Can you work these out from the drawing? Everything is in mm from the part's minimum corner. Give positions to 0.01 mm unless a question says otherwise; leave off trailing zeros. Order: outer loops, then holes, each group sorted by start corner. A loop starts at its lowest first (then second) coordinate and runs counter-clockwise, first axis right, second up. Notation, with made-up numbers: M -37.75,47.25 L -9.75,47.25 A19 cw -9.75,69.25 Z; hole C 28.5,61.5 d7. An arc over 180 degrees is marked long. Use a Markdown table: item, result. Add a question column.
Item 1: Suppose I cut it at B-B on y = 12. Write out the boundary of the cut face in (x, z).
Item 2: If we mould it in two halves opening along Z, with no side actions, what happens to the marked faces 1, 2 and 3? For each: released by +Z, released by -Z, zero draft, split by the parting line, or undercut.
Item 3: If I drill on L1, parallel to Y at x = 3.6, z = 35.5 (1 decimal); L2, parallel to Y at x = 3.25, z = 20; L3, parallel to Z at x = 4.4, y = 7.5 (1 decimal), over which ranges is the centre line in solid material (lowest first)? Write a range as from..to.
Item 4: Suppose I cut it at D-D on x = 2.15. Write out the boundary of the cut face in (y, z).
Item 5: Suppose I cut it at C-C on z = 4. Write out the boundary of the cut face in (x, y), plus the area to 3 significant figures.
Item 6: Suppose I cut it at A-A on z = 20. Write out the boundary of the cut face in (x, y).
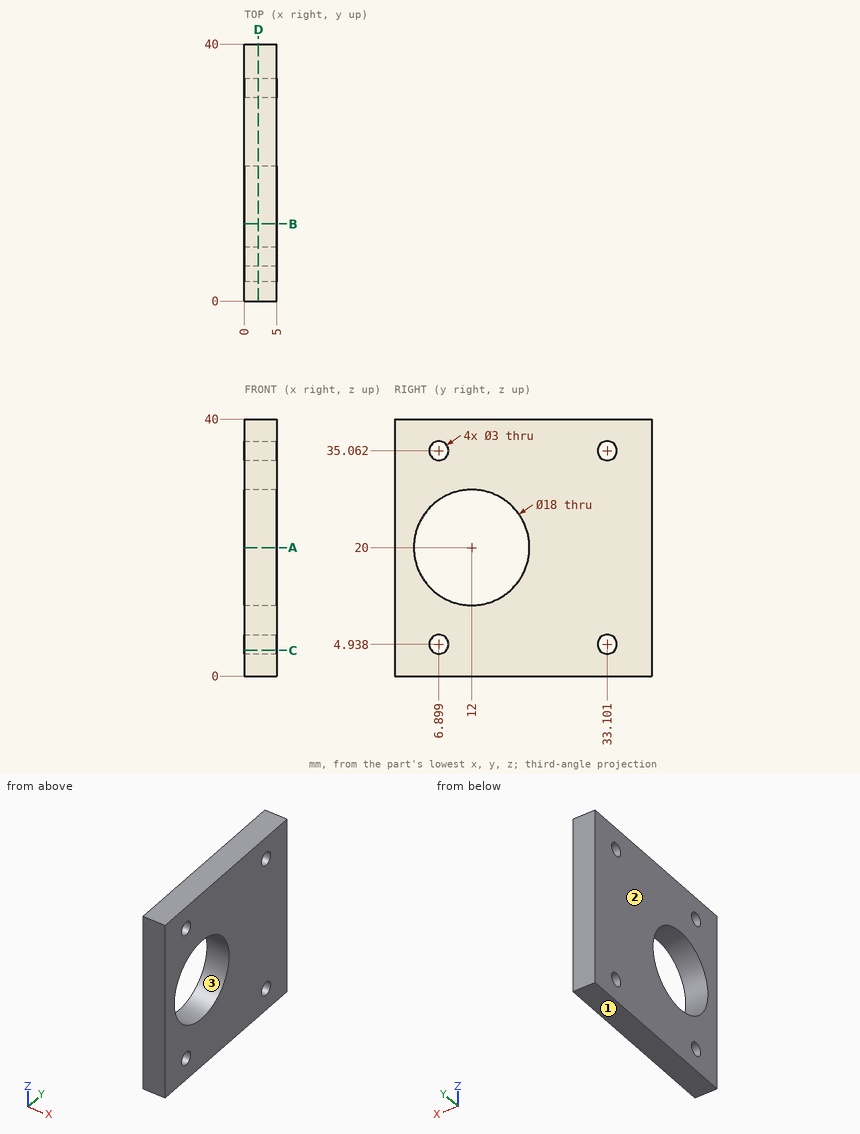
Findings below:
| question | item | result |
|---|---|---|
| 1 | outline | M 0,0 L 5,0 L 5,11 L 0,11 Z; M 0,29 L 5,29 L 5,40 L 0,40 Z |
| 2 | face 1 | released by -Z |
| 2 | face 2 | zero draft |
| 2 | face 3 | undercut |
| 3 | L1 | y = 0..5.5, 8.3..31.7, 34.5..40 |
| 3 | L2 | y = 0..3, 21..40 |
| 3 | L3 | z = 0..3.6, 6.3..12.2, 27.8..33.7, 36.4..40 |
| 4 | outline | M 0,0 L 40,0 L 40,40 L 0,40 Z; hole C 12,20 d18; hole C 6.9,4.94 d3; hole C 6.9,35.06 d3; hole C 33.1,4.94 d3; hole C 33.1,35.06 d3 |
| 5 | outline | M 0,0 L 5,0 L 5,5.73 L 0,5.73 Z; M 0,8.07 L 5,8.07 L 5,31.93 L 0,31.93 Z; M 0,34.27 L 5,34.27 L 5,40 L 0,40 Z |
| 5 | area | 177 mm^2 |
| 6 | outline | M 0,0 L 5,0 L 5,3 L 0,3 Z; M 0,21 L 5,21 L 5,40 L 0,40 Z |
